Source: CAD feature listing. Evaluate the final solid. Frame: model axes, mm. A direction names the side the tool comes from. Give positions to 0.01 mm unless a question says otherwise; leave off trailing zeros. Order: outer loops, then holes, each group sorted by start corner. A loop starts at its lowest first (then second) coordinate and runs counter-clockwise, first axis right, second up.
```python
from build123d import *

# Parameters (mm, degrees)
SKETCH_R             = 1.6
PAD_DEPTH            = 42
SKETCH001_R          = 1.65
POCKET_DEPTH         = 7.001
POCKET_DEPTH_BACK    = 12.001
POCKET001_DEPTH      = 26.001
POCKET001_DEPTH_BACK = 21.001
POCKET002_DEPTH      = 3.5
CHAMFER_ANGLE        = 69.184
CHAMFER_SIZE         = 0.35
SKETCH004_R          = 3.1
POCKET003_DEPTH      = 2
SKETCH005_R          = 12
POCKET004_DEPTH      = 12.001


with BuildPart() as part:
    # Sketch → Pad (new body)
    with BuildSketch(Plane.XZ):
        Polygon((-26, -7), (21, -7), (21, 0), (11, 0), (11, 5.85), (4.85, 12), (-21.85, 12), (-26, 7.85), align=None)
        with Locations((-19, 6)):
            Circle(SKETCH_R, mode=Mode.SUBTRACT)
        with Locations((3, 6)):
            Circle(SKETCH_R, mode=Mode.SUBTRACT)
    extrude(amount=-PAD_DEPTH)

    # Sketch001 → Pocket (cut, two sides)
    with BuildSketch(Plane.XY) as pocket_sk:
        with Locations((-15.5, 36.5)):
            Circle(SKETCH001_R)
        with Locations((15.5, 5.5)):
            Circle(SKETCH001_R)
        with BuildLine():
            Line((-27, 31.35), (-15.35, 43))
            Line((-15.35, 43), (-14.5, 43))
            Line((-14.5, 43), (-11, 39.5))
            Line((-11, 39.5), (-11, 24.354102))
            ThreePointArc((-11, 24.354102), (-1.447855, 9.591507), (11.489125, 21.5))
            Line((11.489125, 21.5), (16, 21.5))
            Line((16, 21.5), (22, 15.5))
            Line((22, 15.5), (22, 44))
            Line((22, 44), (-27, 44))
            Line((-27, 44), (-27, 31.35))
        make_face()
        Polygon((21.5, 2), (19.5, 0), (21.5, 0), align=None)
    extrude(amount=-POCKET_DEPTH, mode=Mode.SUBTRACT)
    extrude(pocket_sk.sketch, amount=POCKET_DEPTH_BACK, mode=Mode.SUBTRACT)

    # Sketch002 → Pocket001 (cut, two sides)
    with BuildSketch(Plane.YZ) as pocket001_sk:
        Polygon((7, 13), (7, 1.785529), (9.55, 0), (43, 0), (43, 13), align=None)
        Polygon((0, -7.3), (1, -7.3), (0, -6.3), align=None)
    extrude(amount=-POCKET001_DEPTH, mode=Mode.SUBTRACT)
    extrude(pocket001_sk.sketch, amount=POCKET001_DEPTH_BACK, mode=Mode.SUBTRACT)

    # Sketch003 (on Face18 of Pocket001) → Pocket002 (cut)
    with BuildSketch(Plane(origin=(0, 7, 0), x_dir=(1, 0, 0), z_dir=(0, 1, 0))):
        Polygon((-16.315, -4.449815), (-19, -2.899629), (-21.685, -4.449815), (-21.685, -7.550185), (-19, -9.100371), (-16.315, -7.550185), align=None)
        Polygon((5.685, -4.449815), (3, -2.899629), (0.315, -4.449815), (0.315, -7.550185), (3, -9.100371), (5.685, -7.550185), align=None)
    extrude(amount=-POCKET002_DEPTH, mode=Mode.SUBTRACT)

    # Chamfer
    chamfer_edges = [part.edges().sort_by_distance(p)[0] for p in [
        (-16.315, 7, 6),
        (-17.6575, 7, 3.674722),
        (-20.3425, 7, 3.674722),
        (-21.685, 7, 6),
        (-20.3425, 7, 8.325278),
        (-17.6575, 7, 8.325278),
        (1.6575, 7, 8.325278),
        (4.3425, 7, 8.325278),
        (5.685, 7, 6),
        (4.3425, 7, 3.674722),
        (1.6575, 7, 3.674722),
        (0.315, 7, 6),
    ]]
    chamfer_side = part.faces().sort_by_distance((-7.961685, 7, 6.742023))[0]
    chamfer(chamfer_edges, length=CHAMFER_SIZE, angle=CHAMFER_ANGLE, reference=chamfer_side)

    # Sketch004 (on Face28 of Chamfer) → Pocket003 (cut)
    with BuildSketch(Plane(origin=(0, 0, 0), x_dir=(-1, 0, 0), z_dir=(0, 0, 1))):
        with Locations((-15.5, -5.5)):
            Circle(SKETCH004_R)
        with Locations((15.5, -36.5)):
            Circle(SKETCH004_R)
    extrude(amount=-POCKET003_DEPTH, mode=Mode.SUBTRACT)

    # Sketch005 → Pocket004 (cut, through all)
    with BuildSketch(Plane.XY):
        with Locations((0, 21)):
            Circle(SKETCH005_R)
    extrude(amount=POCKET004_DEPTH, mode=Mode.SUBTRACT)


solid = part.part
```
1) Section query B-B, the plane y = 12.5. Return the cut outline in (x, z), and give its area (3 significant figures).
Report:
outline: (-26, -7) - (-7.75, -7) - (-7.75, 0) - (-26, 0) - close; (7.75, -7) - (21, -7) - (21, 0) - (7.75, 0) - close
area: 221 mm2
2) Material intervals for L1, parallel to Y at x = 15.5, z = -4.75; L2, parallel to Y at x = -15.5, z = -0.45; L3, parallel to Z at x = -19, y = 2, sorted ascending.
Report:
L1: y = 0 to 3.85, 7.15 to 21.5
L2: y = 0 to 33.4, 39.6 to 42
L3: z = -7 to 4.4, 7.6 to 12
3) Section query D-D, the plane y = 36.5. Return the cut outline in (x, z).
Report:
outline: (-21.85, -7) - (-17.15, -7) - (-17.15, -2) - (-18.6, -2) - (-18.6, 0) - (-21.85, 0) - close; (-13.85, -7) - (-11, -7) - (-11, 0) - (-12.4, 0) - (-12.4, -2) - (-13.85, -2) - close
4) Section query A-A, the plane y = 5.5. Return the cut outline in (x, z) (3 decimals).
Report:
outline: (-26, -7) - (13.85, -7) - (13.85, -2) - (12.4, -2) - (12.4, 0) - (11, 0) - (11, 5.85) - (4.85, 12) - (-21.85, 12) - (-26, 7.85) - close; (17.15, -7) - (21, -7) - (21, 0) - (18.6, 0) - (18.6, -2) - (17.15, -2) - close; hole (-21.685, 4.45) - (-19, 2.9) - (-16.315, 4.45) - (-16.315, 7.55) - (-19, 9.1) - (-21.685, 7.55) - close; hole (0.315, 4.45) - (3, 2.9) - (5.685, 4.45) - (5.685, 7.55) - (3, 9.1) - (0.315, 7.55) - close
5) Reachability of faces 4 (the flat face through (5.685, 5, 6)), 5 (the flat face through (-26, 12, -1)), 6 (the flat face through (-11, 32, -3)) from +Z, -Z, +X, -X, +Y, -Y: full face, straight path, thin tool, end or side. Return the list, or none.
Report:
face 4: +Y
face 5: +Z, -Z, -X, +Y, -Y
face 6: +Z, -Z, +X, +Y
6) Draft query along Z for faces 1 (the flat face through (4.45, 6.53, 3.54)), 2 (the flat face through (-17, 38, -2)), 3 (the cylindrical face through (-1.73, 9.63, -3.45)). Return one class per face: +Z half, -Z half, draft (parallel to the pull), parting line (faces both ways), or undercut.
Report:
face 1: undercut
face 2: +Z half
face 3: draft
7) Section query C-C, the plane x = -8.5. Return the cut outline in (y, z).
Report:
outline: (0, -6.3) - (0.7, -7) - (13.25, -7) - (13.25, 0) - (9.55, 0) - (7, 1.79) - (7, 12) - (0, 12) - close
8) Pin query (flat end, axial travel): pin 1 (0.8 mm diameter, centred on y = 5.5, z = 6, fed in from +X); pin 2 (6 mm diameter, centred on x = 0.5, z = -2, fed in from +Y); pin 3 (8 mm diameter, centred on x = 14.5, z = 6, fed in from +Y). Return the tip coordinate at first contact, or that it passes through.
Report:
pin 1: stops at x = 11
pin 2: stops at y = 10.05
pin 3: stops at y = 7
